CAD build for the part. Positions are in the model's coordinates, mm. Face numbers are marked on the shaded views. A direction names the side the tool comes from. Give positions to 0.01 mm unless a question says otherwise; leave off trailing zeros. Loops run counter-clockwise (first coordinate to the right, second up) from the corner with the lowest first, then second, coordinate; pieces in that order, holes last. Notation, with made-up numbers: M 43,81.25 L 102,81.25 A8 cw 102,91.25 Z; hole C 57,-5 d5. An arc over 180 degrees is marked long. One line per question, with ' | ' between items.
```python
from build123d import *

# Parameters (mm, degrees)
SKETCH_W        = 120
SKETCH_H        = 60
PAD_DEPTH       = 35
POCKET_DEPTH    = 60.001
SKETCH002_W     = 15
SKETCH002_H     = 15
PAD001_DEPTH    = 35
SKETCH003_R     = 10
POCKET001_DEPTH = 35.001
SKETCH004_W     = 60
SKETCH004_H     = 60
POCKET002_DEPTH = 10


with BuildPart() as part:
    # Sketch → Pad (new body)
    with BuildSketch(Plane.XY):
        Rectangle(SKETCH_W, SKETCH_H)
    extrude(amount=PAD_DEPTH)

    # Sketch001 → Pocket (cut, through all)
    with BuildSketch(Plane.XZ.offset(30)):
        Polygon((-45, 35), (-45, 25), (60, 15), (60, 35), align=None)
    extrude(amount=-POCKET_DEPTH, mode=Mode.SUBTRACT)

    # Sketch002 → Pad001 (new body)
    with BuildSketch(Plane(origin=(0, 0, 0), x_dir=(1, 0, 0), z_dir=(0, 0, -1))):
        with Locations((52.5, 22.5)):
            Rectangle(SKETCH002_W, SKETCH002_H)
        with Locations((52.5, -22.5)):
            Rectangle(SKETCH002_W, SKETCH002_H)
    extrude(amount=-PAD001_DEPTH)

    # Sketch003 → Pocket001 (cut, through all)
    with BuildSketch(Plane(origin=(0, 0, 0), x_dir=(1, 0, 0), z_dir=(0, 0, -1))):
        with Locations((-22.5, 0)):
            Circle(SKETCH003_R)
        with Locations((22.5, 0)):
            Circle(SKETCH003_R)
    extrude(amount=-POCKET001_DEPTH, mode=Mode.SUBTRACT)

    # Sketch004 → Pocket002 (cut)
    with BuildSketch(Plane(origin=(0, 0, 0), x_dir=(1, 0, 0), z_dir=(0, 0, -1))):
        with Locations((30, 0)):
            Rectangle(SKETCH004_W, SKETCH004_H)
    extrude(amount=-POCKET002_DEPTH, mode=Mode.SUBTRACT)


solid = part.part
```
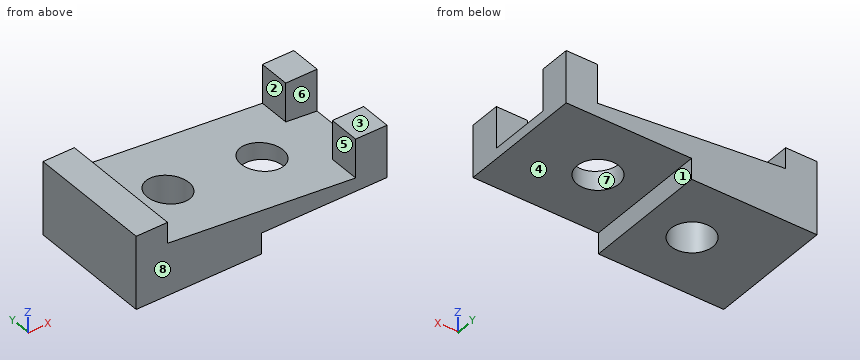
Item 1: Saw through at D-D on z = 5.5. Give the cut face in (x, y), and give its area (3 significant figures).
Conclusion:
outline: M -60,-30 L 0,-30 L 0,30 L -60,30 Z; hole C -22.5,0 d20 | area: 3,290 mm²
Item 2: Saw through at A-A on z = 31. Give the cut face in (x, y), and give its area (3 significant figures).
Conclusion:
outline: M -60,-30 L -45,-30 L -45,30 L -60,30 Z; M 45,-30 L 60,-30 L 60,-15 L 45,-15 Z; M 45,15 L 60,15 L 60,30 L 45,30 Z | area: 1,350 mm²
Item 3: Mould opens along X. For the marked faces 1, 2 and 3 say: pulls with the +X half, pulls with the -X half, needs draft (parallel to the pull), parting line crosses it, or undercut.
Conclusion:
face 1: pulls with the +X half | face 2: undercut | face 3: needs draft
Item 4: Drop flat-ended pins along their axis: P1, Ø3, axis at x = 33, y = 7, coming from the +Z side; P2, Ø6, axis at x = 41.5, z = 21, coming from the -Y side; P3, Ø8, axis at y = 5, z = 27.5, coming from the +X side; P4, Ø8, axis at y = -3.5, z = 5, coming from the +X side. Give the stop position or say it passes through.
Conclusion:
P1: z = 17.71 | P2: through | P3: x = -30.52 | P4: x = 0
Item 5: Saw through at B-B on x = -29. Give the cut face in (y, z).
Conclusion:
outline: M -30,0 L -7.6,0 L -7.6,23.48 L -30,23.48 Z; M 7.6,0 L 30,0 L 30,23.48 L 7.6,23.48 Z
Item 6: Drill centre lines: line 1 along X through (y, z) = (0, 17.75); line 2 along X through (y, z) = (-5.5, 10.5); line 3 along X through (y, z) = (0, 14). Where is each one in solid material? Low to high. Write a range as [from, to].
Conclusion:
line 1: [-60, -32.5], [-12.5, 12.5] | line 2: [-60, -30.85], [-14.15, 14.15], [30.85, 60] | line 3: [-60, -32.5], [-12.5, 12.5], [32.5, 60]
Item 7: Saw through at C-C on y = 5. Give the cut face in (x, z), and give its area (3 significant figures).
Conclusion:
outline: M -60,0 L -31.16,0 L -31.16,23.68 L -45,25 L -45,35 L -60,35 Z; M -13.84,0 L 0,0 L 0,10 L 13.84,10 L 13.84,19.4 L -13.84,22.03 Z; M 31.16,10 L 60,10 L 60,15 L 31.16,17.75 Z | area: 1,480 mm²
Item 8: 3-axis set-ups, long thin cutter, end or side, ignore diameter. For the marked faces 4, 5, 6, 7 and 8: which of +Z, -Z, +X, -X, +Y, -Y reach the whole face in a straight line?
Conclusion:
face 4: -Z, +X, +Y, -Y | face 5: +Z, +Y, -Y | face 6: +Z, +X | face 7: +Z, -Z | face 8: +Z, -Z, +X, -X, -Y
